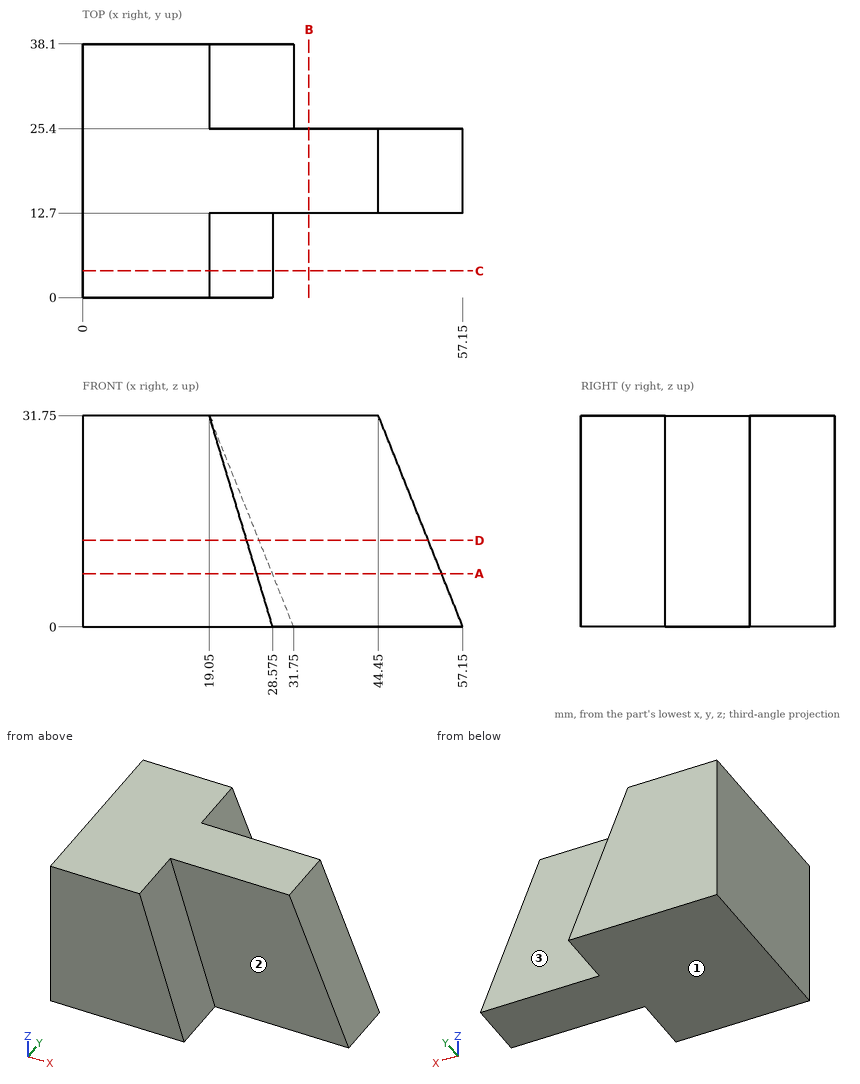
The drawing under review shows one solid part. Ordinate dimensions are in mm from its lowest x, y, z. A direction names the side the tool comes from. Coordinates: 2 decimals unless noted, no trailing zeros. Order: outer loops, then holes, each group sorted by start corner. A loop starts at its lowest first (then second) coordinate and runs counter-clockwise, first axis right, second up. Notation, with made-up numbers: (-11.5, 73) -> (36.5, 73) arc R21 cw to (36.5, 101) -> close; hole circle Ø7 at (82.25, 73.25). An arc over 180 degrees is marked (long way). Answer as CSV lines item,"result".
Q1. For the marked faces 1, 2 and 3, list the 3-axis set-ups (+Z, -Z, +X, -X, +Y, -Y) from which the entire face can be reached by the end or side of a thin tool; tool diameter is ignored.
Model answer:
face 1,"-Z, +X, -X, +Y, -Y"
face 2,"+Z, +X, -Y"
face 3,"+Z, +X, +Y"
Q2. We need section C-C (y = 4). State the section outline as (x, z) points (3 decimals), plus the area to 3 significant figures.
Model answer:
outline,"(0, 0) -> (28.575, 0) -> (19.05, 31.75) -> (0, 31.75) -> close"
area,"756 mm2"
Q3. We need section A-A (z = 8). State the section outline as (x, y) points (3 decimals).
Model answer:
outline,"(0, 0) -> (26.175, 0) -> (26.175, 12.7) -> (53.95, 12.7) -> (53.95, 25.4) -> (28.55, 25.4) -> (28.55, 38.1) -> (0, 38.1) -> close"
Q4. We need section D-D (z = 13). State the section outline as (x, y) points (3 decimals), plus the area to 3 significant figures.
Model answer:
outline,"(0, 0) -> (24.675, 0) -> (24.675, 12.7) -> (51.95, 12.7) -> (51.95, 25.4) -> (26.55, 25.4) -> (26.55, 38.1) -> (0, 38.1) -> close"
area,"1,310 mm2"
Q5. Wall thickness on line 1 along Y through (x, z) = (32.5, 1); line 2 along X through (y, z) = (13.5, 25); line 3 along X through (y, z) = (23, 26): over which ranges is each line inside the solid? List them lowest first. Write a range as [from, to].
Model answer:
line 1,"y = [12.7, 25.4]"
line 2,"x = [0, 47.15]"
line 3,"x = [0, 46.75]"
Q6. Clearance check with flat-ended pins moving along their axes: pin 1 Ø10 at (x, z) = (45, 14) entering from -Y; pin 2 Ø8 at (x, z) = (41.5, 23) entering from +Y; pin 3 Ø1 at (x, z) = (49, 26) entering from -Y; pin 4 Ø1.5 at (y, z) = (13, 4) entering from +X. State where each tip first meets the part, or that it passes through.
Model answer:
pin 1,"stops at y = 12.7"
pin 2,"stops at y = 25.4"
pin 3,"passes through"
pin 4,"stops at x = 55.85"
Q7. We need section B-B (x = 34). State the section outline as (y, z) points.
Model answer:
outline,"(12.7, 0) -> (25.4, 0) -> (25.4, 31.75) -> (12.7, 31.75) -> close"
